Autodesk Inventor part; units mm, degrees
ref_plane "YZ Plane" through (0, 0, 0) normal (1, 0, 0) x (0, 1, 0)
ref_plane "XZ Plane" through (0, 0, 0) normal (0, 1, 0) x (-1, 0, 0)
ref_plane "XY Plane" through (0, 0, 0) normal (0, 0, 1) x (1, 0, 0)
sketch "Sketch1" plane through (0, 0, 0) normal (1, 0, 0) x (0, 1, 0)
  circle A0 centre (0, 0) radius 12.2
  circle A1 centre (0, 0) radius 12.5
  dimension "d0" = 24.4
  dimension "d1" = 25
extrude "Extrusion1" add sketch "Sketch1" along normal blind 31 contours A0
extrude "Extrusion2" add sketch "Sketch1" against normal blind 21 contours A0 | A1
sketch "Sketch2" plane through (-21, 0, 0) normal (-1, 0, 0) x (0, 0, 1)
  circle A0 centre (0, 0) radius 3.5
  dimension "d6" = 7
extrude "Extrusion3" add sketch "Sketch2" along normal blind 2.5
sketch "Sketch3" plane through (-23.5, 0, 0) normal (-1, 0, 0) x (0, 0, 1)
  circle A0 centre (0, 0) radius 2
  dimension "d9" = 4
extrude "Extrusion4" add sketch "Sketch3" along normal blind 9.5
sketch "Sketch4" plane through (-33, 0, 0) normal (-1, 0, 0) x (0, 0, 1)
  circle A0 centre (0, 0) radius 2
  circle A1 centre (0, 0) radius 2
  line L0 (-1.3229, 1.5) -> (1.3229, 1.5)
  circle A2 centre (0, 0) radius 2
  dimension "d12" = 4
  dimension "d13" = 3.5
extrude "Extrusion5" cut sketch "Sketch4" against normal blind 8 contours L0 A0 picked at (-0.3089, 1.5908)
sketch "Sketch5" plane through (-21, 0, 0) normal (-1, 0, 0) x (0, 0, 1)
  arc A0 (-1.3229, 1.5) -> (1.3229, 1.5) centre (0, 0) ccw
  line L0 (0, 0) -> (0, 8.5) construction
  circle A1 centre (0, 8.5) radius 1.25
  line L1 (0, 0) -> (0, -8.5) construction
  circle A2 centre (0, -8.5) radius 1.25
  dimension "d16" = 8.5
  dimension "d17" = 2.5
  dimension "d18" = 8.5
  dimension "d19" = 2.5
extrude "Extrusion6" cut sketch "Sketch5" against normal blind 8
thread "Thread1"
thread "Thread2"
properties part number "motor6kg"
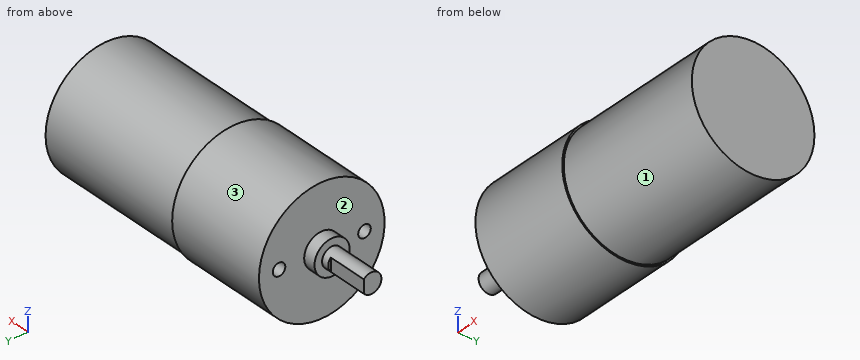
Input: part model. Units: mm. Frame: model coordinates. Face numbers are marked on the shaded views. A direction names the side the tool comes from. Round coordinates to 2 decimals unless told otherwise and drop trailing zeros. Loops run counter-clockwise (first coordinate to the right, second up) from the corner with the lowest first, then second, coordinate; pieces in that order, holes last. Notation, with made-up numbers: (13, -17.5) - (31, -17.5) arc R20 ccw to (31, -8.5) - close; hole circle Ø8 at (26.5, -16.5). An arc over 180 degrees is marked (long way). One line per item, written item: value. Start each with the question number.
(1) Section C-C, the plane x = -16.5. Return loops of the section in (y, z), plus the area to 3 significant figures.
(2) Section B-B, the plane z = 0. Return loops of the section in (x, y).
(3) Section D-D, the plane x = 5. Return loops of the section in (y, z), plus the area to 3 significant figures.
(4) Section A-A, the plane y = 0. Return loops of the section in (x, z), plus the area to 3 significant figures.
(5) Access query for the marked faces 1, 2 and 3. Directions: +Z, -Z, +X, -X, +Y, -Y. A direction counts if a zero-diameter tool reaches every point of the face in a straight line with its end or side. Return the directions, or none.
(6) Ray query, line 1 (X direction, y = 0.5, z = 5.5); line 2 (X direction, y = -9.25, z = -0.5); line 3 (Y direction, x = -2, z = -1.5). Return the intervals inside material, ascending. Write a range as [from, to].
(7) Contact query for flat-ended pins moving along their axis: P1, Ø0.8, axis at y = 8, z = -0.5, coming from the -X side; P2, Ø8, axis at x = -26, y = -6, coming from the -Z side; P3, Ø1.5, axis at x = -5.5, y = 8, coming from the +Z side. Output: stop coordinate, or through.
Results below:
1. outline: circle Ø25 at (0, 0); hole circle Ø2.5 at (-8.5, 0); hole circle Ø2.5 at (8.5, 0)
1. area: 481 mm^2
2. outline: (-33, -2) - (-23.5, -2) - (-23.5, -3.5) - (-21, -3.5) - (-21, -7.25) - (-13, -7.25) - (-13, -9.75) - (-21, -9.75) - (-21, -12.5) - (0, -12.5) - (0, -12.2) - (31, -12.2) - (31, 12.2) - (0, 12.2) - (0, 12.5) - (-21, 12.5) - (-21, 9.75) - (-13, 9.75) - (-13, 7.25) - (-21, 7.25) - (-21, 3.5) - (-23.5, 3.5) - (-23.5, 2) - (-25, 2) - (-25, 1.5) - (-33, 1.5) - close
3. outline: circle Ø24.4 at (0, 0)
3. area: 468 mm^2
4. outline: (-33, -2) - (-23.5, -2) - (-23.5, -3.5) - (-21, -3.5) - (-21, -12.5) - (0, -12.5) - (0, -12.2) - (31, -12.2) - (31, 12.2) - (0, 12.2) - (0, 12.5) - (-21, 12.5) - (-21, 3.5) - (-23.5, 3.5) - (-23.5, 2) - (-33, 2) - close
4. area: 1,340 mm^2
5. face 1: +X
5. face 2: -X
5. face 3: +X, -X
6. line 1: [-21, 31]
6. line 2: [-13, 31]
6. line 3: [-12.41, 12.41]
7. P1: x = -13
7. P2: z = -1.99
7. P3: z = 10.18
